The model under review builds one solid part; all positions refer to its coordinate system, in mm. A direction names the side the tool comes from. Coordinates: 2 decimals unless noted, no trailing zeros. Write each loop counter-clockwise with the first axis right and the second up, starting at its lowest first coordinate (ties: lowest second). Pieces come first, ordered by that corner, then holes. Notation, with made-up numbers: M 71,56 L 116,56 A21 ccw 116,95 Z; hole C 62,42.5 d10. An arc over 180 degrees is marked long. Answer as a JSON object with one key per item and string values.
```python
from build123d import *

# Parameters (mm, degrees)
EXTRUDE_1_DEPTH        = 4
SKETCH_1_4_OUTSIDE_W   = 503.8
SKETCH_1_4_OUTSIDE_H   = 503.8
SKETCH_1_4_OUTSIDE_R   = 1.55
SKETCH_1_4_OUTSIDE_W_2 = 25.4
SKETCH_1_4_OUTSIDE_H_2 = 68.58
SKETCH_1_4_OUTSIDE_H_3 = 15
CUT_EXTRUDE_2_DEPTH    = 4


with BuildPart() as part:
    # Sketch 1 → Extrude 1 (new body)
    with BuildSketch(Plane(origin=(0, 0, 0), x_dir=(1, 0, 0), z_dir=(0, 1, 0))):
        with BuildLine():
            Line((139.7, -195.58), (89.408, -195.58))
            ThreePointArc((89.408, -195.58), (0, -106.172), (-89.408, -195.58))
            Line((-89.408, -195.58), (-139.7, -195.58))
            Line((-139.7, -195.58), (-195.58, -139.7))
            Line((-195.58, -139.7), (-195.58, 139.7))
            Line((-195.58, 139.7), (-139.7, 195.58))
            Line((-139.7, 195.58), (-63.5, 195.58))
            Line((-63.5, 195.58), (-38.1, 106.68))
            Line((-38.1, 106.68), (38.1, 106.68))
            Line((38.1, 106.68), (63.5, 195.58))
            Line((63.5, 195.58), (139.7, 195.58))
            Line((139.7, 195.58), (195.58, 139.7))
            Line((195.58, 139.7), (195.58, -139.7))
            Line((195.58, -139.7), (139.7, -195.58))
        make_face()
    extrude(amount=EXTRUDE_1_DEPTH)

    # Sketch 1_4 outside → Cut-Extrude 2 (cut)
    # profile 1 of 35: a face of its own
    with BuildSketch(Plane(origin=(0, 0, 0), x_dir=(1, 0, 0), z_dir=(0, 1, 0))):
        Rectangle(SKETCH_1_4_OUTSIDE_W, SKETCH_1_4_OUTSIDE_H)
        with BuildLine():
            Line((139.7, -195.58), (89.408, -195.58))
            ThreePointArc((89.408, -195.58), (0, -106.172), (-89.408, -195.58))
            Line((-89.408, -195.58), (-139.7, -195.58))
            Line((-139.7, -195.58), (-195.58, -139.7))
            Line((-195.58, -139.7), (-195.58, 139.7))
            Line((-195.58, 139.7), (-139.7, 195.58))
            Line((-139.7, 195.58), (-63.5, 195.58))
            Line((-63.5, 195.58), (-38.1, 106.68))
            Line((-38.1, 106.68), (38.1, 106.68))
            Line((38.1, 106.68), (63.5, 195.58))
            Line((63.5, 195.58), (139.7, 195.58))
            Line((139.7, 195.58), (195.58, 139.7))
            Line((195.58, 139.7), (195.58, -139.7))
            Line((195.58, -139.7), (139.7, -195.58))
        make_face(mode=Mode.SUBTRACT)
    # profile 2 of 35: a face of its own
    with BuildSketch(Plane(origin=(0, 0, 0), x_dir=(1, 0, 0), z_dir=(0, 1, 0))):
        with Locations(Location((-83.566, 139.7, 0), (0, 0, 270))):
            Circle(SKETCH_1_4_OUTSIDE_R)
    # profile 3 of 35: a face of its own
    with BuildSketch(Plane(origin=(0, 0, 0), x_dir=(1, 0, 0), z_dir=(0, 1, 0))):
        with Locations(Location((-129.286, 139.7, 0), (0, 0, 270))):
            Circle(SKETCH_1_4_OUTSIDE_R)
    # profile 4 of 35: a face of its own
    with BuildSketch(Plane(origin=(0, 0, 0), x_dir=(1, 0, 0), z_dir=(0, 1, 0))):
        with Locations(Location((-83.566, -106.68, 0), (0, 0, 270))):
            Circle(SKETCH_1_4_OUTSIDE_R)
    # profile 5 of 35: a face of its own
    with BuildSketch(Plane(origin=(0, 0, 0), x_dir=(1, 0, 0), z_dir=(0, 1, 0))):
        with Locations(Location((-129.286, -106.68, 0), (0, 0, 270))):
            Circle(SKETCH_1_4_OUTSIDE_R)
    # profile 6 of 35: a face of its own
    with BuildSketch(Plane(origin=(0, 0, 0), x_dir=(1, 0, 0), z_dir=(0, 1, 0))):
        with Locations(Location((83.566, 139.7, 0), (0, 0, 270))):
            Circle(SKETCH_1_4_OUTSIDE_R)
    # profile 7 of 35: a face of its own
    with BuildSketch(Plane(origin=(0, 0, 0), x_dir=(1, 0, 0), z_dir=(0, 1, 0))):
        with Locations(Location((129.286, 139.7, 0), (0, 0, 270))):
            Circle(SKETCH_1_4_OUTSIDE_R)
    # profile 8 of 35: a face of its own
    with BuildSketch(Plane(origin=(0, 0, 0), x_dir=(1, 0, 0), z_dir=(0, 1, 0))):
        with Locations(Location((83.566, -106.68, 0), (0, 0, 270))):
            Circle(SKETCH_1_4_OUTSIDE_R)
    # profile 9 of 35: a face of its own
    with BuildSketch(Plane(origin=(0, 0, 0), x_dir=(1, 0, 0), z_dir=(0, 1, 0))):
        with Locations(Location((129.286, -106.68, 0), (0, 0, 270))):
            Circle(SKETCH_1_4_OUTSIDE_R)
    # profile 10 of 35: a face of its own
    with BuildSketch(Plane(origin=(0, 0, 0), x_dir=(1, 0, 0), z_dir=(0, 1, 0))):
        with Locations(Location((-129.286, 71.12, 0), (0, 0, 270))):
            Circle(SKETCH_1_4_OUTSIDE_R)
    # profile 11 of 35: a face of its own
    with BuildSketch(Plane(origin=(0, 0, 0), x_dir=(1, 0, 0), z_dir=(0, 1, 0))):
        with Locations(Location((-83.566, 71.12, 0), (0, 0, 270))):
            Circle(SKETCH_1_4_OUTSIDE_R)
    # profile 12 of 35: a face of its own
    with BuildSketch(Plane(origin=(0, 0, 0), x_dir=(1, 0, 0), z_dir=(0, 1, 0))):
        with Locations(Location((83.566, 71.12, 0), (0, 0, 270))):
            Circle(SKETCH_1_4_OUTSIDE_R)
    # profile 13 of 35: a face of its own
    with BuildSketch(Plane(origin=(0, 0, 0), x_dir=(1, 0, 0), z_dir=(0, 1, 0))):
        with Locations(Location((129.286, 71.12, 0), (0, 0, 270))):
            Circle(SKETCH_1_4_OUTSIDE_R)
    # profile 14 of 35: a face of its own
    with BuildSketch(Plane(origin=(0, 0, 0), x_dir=(1, 0, 0), z_dir=(0, 1, 0))):
        with Locations(Location((-129.286, -38.1, 0), (0, 0, 270))):
            Circle(SKETCH_1_4_OUTSIDE_R)
    # profile 15 of 35: a face of its own
    with BuildSketch(Plane(origin=(0, 0, 0), x_dir=(1, 0, 0), z_dir=(0, 1, 0))):
        with Locations(Location((-83.566, -38.1, 0), (0, 0, 270))):
            Circle(SKETCH_1_4_OUTSIDE_R)
    # profile 16 of 35: a face of its own
    with BuildSketch(Plane(origin=(0, 0, 0), x_dir=(1, 0, 0), z_dir=(0, 1, 0))):
        with Locations(Location((83.566, -38.1, 0), (0, 0, 270))):
            Circle(SKETCH_1_4_OUTSIDE_R)
    # profile 17 of 35: a face of its own
    with BuildSketch(Plane(origin=(0, 0, 0), x_dir=(1, 0, 0), z_dir=(0, 1, 0))):
        with Locations(Location((129.286, -38.1, 0), (0, 0, 270))):
            Circle(SKETCH_1_4_OUTSIDE_R)
    # profile 18 of 35: a face of its own
    with BuildSketch(Plane(origin=(0, 0, 0), x_dir=(1, 0, 0), z_dir=(0, 1, 0))):
        with Locations(Location((-178, -38.1, 0), (0, 0, 270))):
            Circle(SKETCH_1_4_OUTSIDE_R)
    # profile 19 of 35: a face of its own
    with BuildSketch(Plane(origin=(0, 0, 0), x_dir=(1, 0, 0), z_dir=(0, 1, 0))):
        with Locations(Location((-178, -106.68, 0), (0, 0, 270))):
            Circle(SKETCH_1_4_OUTSIDE_R)
    # profile 20 of 35: a face of its own
    with BuildSketch(Plane(origin=(0, 0, 0), x_dir=(1, 0, 0), z_dir=(0, 1, 0))):
        with Locations(Location((178, -106.68, 0), (0, 0, 270))):
            Circle(SKETCH_1_4_OUTSIDE_R)
    # profile 21 of 35: a face of its own
    with BuildSketch(Plane(origin=(0, 0, 0), x_dir=(1, 0, 0), z_dir=(0, 1, 0))):
        with Locations(Location((178, -38.1, 0), (0, 0, 270))):
            Circle(SKETCH_1_4_OUTSIDE_R)
    # profile 22 of 35: a face of its own
    with BuildSketch(Plane(origin=(0, 0, 0), x_dir=(1, 0, 0), z_dir=(0, 1, 0))):
        with Locations(Location((-178, 139.7, 0), (0, 0, 270))):
            Circle(SKETCH_1_4_OUTSIDE_R)
    # profile 23 of 35: a face of its own
    with BuildSketch(Plane(origin=(0, 0, 0), x_dir=(1, 0, 0), z_dir=(0, 1, 0))):
        with Locations(Location((-178, 71.12, 0), (0, 0, 270))):
            Circle(SKETCH_1_4_OUTSIDE_R)
    # profile 24 of 35: a face of its own
    with BuildSketch(Plane(origin=(0, 0, 0), x_dir=(1, 0, 0), z_dir=(0, 1, 0))):
        with Locations(Location((178, 139.7, 0), (0, 0, 270))):
            Circle(SKETCH_1_4_OUTSIDE_R)
    # profile 25 of 35: a face of its own
    with BuildSketch(Plane(origin=(0, 0, 0), x_dir=(1, 0, 0), z_dir=(0, 1, 0))):
        with Locations(Location((178, 71.12, 0), (0, 0, 270))):
            Circle(SKETCH_1_4_OUTSIDE_R)
    # profile 26 of 35: a face of its own
    with BuildSketch(Plane(origin=(0, 0, 0), x_dir=(1, 0, 0), z_dir=(0, 1, 0))):
        with Locations(Location((-38.1, 72, 0), (0, 0, 270))):
            Circle(SKETCH_1_4_OUTSIDE_R)
    # profile 27 of 35: a face of its own
    with BuildSketch(Plane(origin=(0, 0, 0), x_dir=(1, 0, 0), z_dir=(0, 1, 0))):
        with Locations(Location((38.1, 72, 0), (0, 0, 270))):
            Circle(SKETCH_1_4_OUTSIDE_R)
    # profile 28 of 35: a face of its own
    with BuildSketch(Plane(origin=(0, 0, 0), x_dir=(1, 0, 0), z_dir=(0, 1, 0))):
        with Locations(Location((-38.1, 19, 0), (0, 0, 270))):
            Circle(SKETCH_1_4_OUTSIDE_R)
    # profile 29 of 35: a face of its own
    with BuildSketch(Plane(origin=(0, 0, 0), x_dir=(1, 0, 0), z_dir=(0, 1, 0))):
        with Locations(Location((38.1, 19, 0), (0, 0, 270))):
            Circle(SKETCH_1_4_OUTSIDE_R)
    # profile 30 of 35: a face of its own
    with BuildSketch(Plane(origin=(0, 0, 0), x_dir=(1, 0, 0), z_dir=(0, 1, 0))):
        with Locations((-149.86, 105.41)):
            Rectangle(SKETCH_1_4_OUTSIDE_W_2, SKETCH_1_4_OUTSIDE_H_2)
    # profile 31 of 35: a face of its own
    with BuildSketch(Plane(origin=(0, 0, 0), x_dir=(1, 0, 0), z_dir=(0, 1, 0))):
        with Locations((149.86, 105.41)):
            Rectangle(SKETCH_1_4_OUTSIDE_W_2, SKETCH_1_4_OUTSIDE_H_2)
    # profile 32 of 35: a face of its own
    with BuildSketch(Plane(origin=(0, 0, 0), x_dir=(1, 0, 0), z_dir=(0, 1, 0))):
        with Locations((149.86, -72.39)):
            Rectangle(SKETCH_1_4_OUTSIDE_W_2, SKETCH_1_4_OUTSIDE_H_2)
    # profile 33 of 35: a face of its own
    with BuildSketch(Plane(origin=(0, 0, 0), x_dir=(1, 0, 0), z_dir=(0, 1, 0))):
        with Locations((-149.86, -72.39)):
            Rectangle(SKETCH_1_4_OUTSIDE_W_2, SKETCH_1_4_OUTSIDE_H_2)
    # profile 34 of 35: a face of its own
    with BuildSketch(Plane(origin=(0, 0, 0), x_dir=(1, 0, 0), z_dir=(0, 1, 0))):
        with Locations((-127, 0)):
            Rectangle(SKETCH_1_4_OUTSIDE_W_2, SKETCH_1_4_OUTSIDE_H_3)
    # profile 35 of 35: a face of its own
    with BuildSketch(Plane(origin=(0, 0, 0), x_dir=(1, 0, 0), z_dir=(0, 1, 0))):
        with Locations((127, 0)):
            Rectangle(SKETCH_1_4_OUTSIDE_W_2, SKETCH_1_4_OUTSIDE_H_3)
    extrude(amount=CUT_EXTRUDE_2_DEPTH, mode=Mode.SUBTRACT)


solid = part.part
```
(1) Draft analysis for pull direction X (two halves, no side actions). For faces 3 (the face through (-167.25, 1.97, 168.03)), 4 (the face through (1.966, 1.972, 106.194)), 5 (the face through (167.25, 1.97, -168.03)), state which applies: released by +X, released by -X, zero draft, split by the parting line, or undercut.
Results list:
{"face 3": "released by -X", "face 4": "undercut", "face 5": "released by +X"}
(2) Add section B-B on x = -17. Give the boundary of the cut face in (y, z), and give its area (3 significant figures).
Results list:
{"outline": "M 0,-106.68 L 4,-106.68 L 4,107.8 L 0,107.8 Z", "area": "858 mm²"}
(3) Add section A-A on z = 171.5. Give the boundary of the cut face in (x, y).
Results list:
{"outline": "M -163.78,0 L -86.1,0 L -86.1,4 L -163.78,4 Z; M 86.1,0 L 163.78,0 L 163.78,4 L 86.1,4 Z"}
(4) Wall thickness on line 1 along X through (y, z) = (1.65, -6.5); line 2 along X through (y, z) = (3.1, 75.5); line 3 along Z through (x, y) = (129.5, 1.45): over which ranges is each line inside the solid? List them lowest first. Write a range as from..to.
Results list:
{"line 1": "-195.58..-139.7, -114.3..114.3, 139.7..195.58", "line 2": "-195.58..-162.56, -137.16..137.16, 162.56..195.58", "line 3": "-195.58..-141.24, -138.16..-72.66, -69.58..-7.5, 7.5..36.56, 39.64..105.14, 108.22..195.58"}
(5) Add section C-C on x = -75. Give the boundary of the cut face in (y, z).
Results list:
{"outline": "M 0,-195.58 L 4,-195.58 L 4,146.91 L 0,146.91 Z"}
(6) For faces 1 (the face through (-168.03, 1.97, -167.25)), 2 (the face through (-50.978, 1.972, -151.752)), list the 3-axis set-ups (+Z, -Z, +X, -X, +Y, -Y) from which the entire face can be reached by the end or side of a thin tool; tool diameter is ignored.
Results list:
{"face 1": "-Z, -X, +Y, -Y", "face 2": "-Z, +Y, -Y"}
(7) For pin 1 Ø3 at (x, z) = (-129.286, 106.68) entering from -Y; pin 2 Ø1.2 at (x, y) = (147, 2.5) entering from +Z, all flat-tipped, find the tip position at first contact; note any pin that passes through.
Results list:
{"pin 1": "through", "pin 2": "z = 188.88"}
